Check sheet for the modelled part. Datum: model origin and axes. Units: mm. Round coordinates to 2 decimals unless told otherwise and drop trailing zeros. Loops run counter-clockwise (first coordinate to the right, second up) from the corner with the lowest first, then second, coordinate; pieces in that order, holes last. Notation, with made-up numbers: (88.25, 8.5) -> (111.25, 8.5) arc R18 ccw to (111.25, 14.5) -> close; hole circle Ø3 at (31, 28.25). An arc over 180 degrees is marked (long way). One line per question, with ' | ' between items.
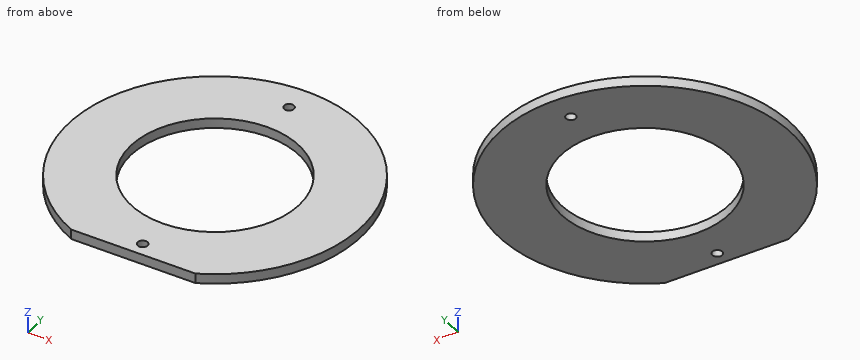
```python
from build123d import *

# Parameters (mm, degrees)
BOSS_EXTRUDE1_DEPTH = 5
SKETCH2_R           = 2.5
CUT_EXTRUDE1_DEPTH  = 10
CUT_EXTRUDE2_REACH  = 225.261
SKETCH3_R           = 42.5


with BuildPart() as part:
    # Sketch1 → Boss-Extrude1 (new body)
    with BuildSketch(Plane.XY):
        with BuildLine():
            Line((-125.81358794, 5.502409601), (-62.980475651, 5.502409601))
            ThreePointArc((-62.980475651, 5.502409601), (-94.397031795, 146.502409601), (-125.81358794, 5.502409601))
        make_face()
    extrude(amount=BOSS_EXTRUDE1_DEPTH)

    # Sketch2 → Cut-Extrude1 (cut)
    with BuildSketch(Plane.XY.offset(5)):
        with Locations((-93.953395264, 132.502409601)):
            Circle(SKETCH2_R)
        with Locations((-93.953395264, 12.502409601)):
            Circle(SKETCH2_R)
    extrude(amount=-CUT_EXTRUDE1_DEPTH, mode=Mode.SUBTRACT)

    # Sketch3 → Cut-Extrude2 (cut, up to next)
    with BuildSketch(Plane.XY.offset(5), mode=Mode.PRIVATE) as cut_extrude2_sk1:
        with Locations((-94.397031795, 72.502409601)):
            Circle(SKETCH3_R)
    cut_extrude2_tool1 = extrude(cut_extrude2_sk1.sketch, amount=-CUT_EXTRUDE2_REACH, mode=Mode.PRIVATE) & part.part
    add(cut_extrude2_tool1.solids().sort_by_distance((-94.397032, 72.50241, 5))[0], mode=Mode.SUBTRACT)


solid = part.part
```
(1) Sectioned sample at C-C, the plane z = 0.9. Record the cut outline in (x, y).
Answer:
outline: (-125.81, 5.5) -> (-62.98, 5.5) arc R74 ccw (long way) to start; hole circle Ø85 at (-94.4, 72.5); hole circle Ø5 at (-93.95, 12.5); hole circle Ø5 at (-93.95, 132.5)
(2) Scan lines: probe 1 along Y at (x, z) = (-92.5, 1.55); probe 2 along X at (y, z) = (95, 2.2); probe 3 along Y at (x, z) = (-97, 1.95). Record each from-to range of solid material in increasing order.
Answer:
probe 1: y = 5.5 to 10.47, 14.54 to 30.04, 114.96 to 130.47, 134.54 to 146.48 | probe 2: x = -164.89 to -130.45, -58.34 to -23.9 | probe 3: y = 5.5 to 30.08, 114.92 to 146.46
(3) Sectioned sample at D-D, the plane x = -31. Record the cut outline in (y, z), and give its area (3 significant figures).
Answer:
outline: (34.33, 0) -> (110.67, 0) -> (110.67, 5) -> (34.33, 5) -> close | area: 382 mm2
(4) Go/stop test with flat-tipped pins: pin 1 (4.5 mm diameter, centred on x = -93.95, y = 132.5, fed in from -Z) (3 decimals); pin 2 (10 mm diameter, centred on x = -146.5, y = 34, fed in from -Z). Record where each tip stops, or that it passes through.
Answer:
pin 1: passes through | pin 2: stops at z = 0
(5) Sectioned sample at B-B, the plane x = -106. Record the cut outline in (y, z).
Answer:
outline: (5.5, 0) -> (31.62, 0) -> (31.62, 5) -> (5.5, 5) -> close; (113.39, 0) -> (145.59, 0) -> (145.59, 5) -> (113.39, 5) -> close
(6) Sectioned sample at A-A, the plane y = 56. Record the cut outline in (x, z).
Answer:
outline: (-166.53, 0) -> (-133.56, 0) -> (-133.56, 5) -> (-166.53, 5) -> close; (-55.23, 0) -> (-22.26, 0) -> (-22.26, 5) -> (-55.23, 5) -> close
